```python
from build123d import *

# Parameters (mm, degrees)
BOSS_EXTRUDE1_DEPTH            = 4
SKETCH2_R                      = 2.2
BOSS_EXTRUDE2_DEPTH            = 3.5
SKETCH3_R                      = 0.75
CUT_EXTRUDE1_DEPTH             = 8.5
SKETCH4_R                      = 2.2
BOSS_EXTRUDE3_DEPTH            = 3.5
SKETCH5_R                      = 0.75
CUT_EXTRUDE2_DEPTH             = 8.5
SKETCH6_R                      = 2.2
BOSS_EXTRUDE4_DEPTH            = 3.5
SKETCH7_R                      = 0.75
CUT_EXTRUDE3_DEPTH             = 8.5
SKETCH8_R                      = 2.2
BOSS_EXTRUDE5_DEPTH            = 3.5
SKETCH9_R                      = 0.75
CUT_EXTRUDE4_DEPTH             = 8.5
SKETCH10_W                     = 20
SKETCH10_H                     = 5
BOSS_EXTRUDE6_DEPTH            = 3.5
SKETCH11_R                     = 1.5
CUT_EXTRUDE5_DEPTH             = 8.5
BOSS_EXTRUDE8_DEPTH            = 5
CBORE_FOR_M3_SHCS1_D           = 3.4
CBORE_FOR_M3_SHCS1_CBORE_D     = 6.5
CBORE_FOR_M3_SHCS1_CBORE_DEPTH = 3
FILLET1_R                      = 5
FILLET2_R                      = 3


with BuildPart() as part:
    # Sketch1 → Boss-Extrude1 (new body)
    with BuildSketch(Plane.XY):
        with BuildLine():
            Line((0, 0), (59.790168207, -3.934842784))
            ThreePointArc((59.790168207, -3.934842784), (63.68729409, -6.932891166), (62.399590235, -11.678173352))
            Line((62.399590235, -11.678173352), (40.5, -28.758482209))
            Line((40.5, -28.758482209), (40.5, -46.843965811))
            Line((40.5, -46.843965811), (35.5, -46.843965811))
            Line((35.5, -46.843965811), (35.5, -23.843965811))
            Line((35.5, -23.843965811), (23, -23.843965811))
            Line((23, -23.843965811), (23, -9.315581275))
            Line((23, -9.315581275), (-23, -9.315581275))
            Line((-23, -9.315581275), (-23, -23.843965815))
            Line((-23, -23.843965815), (-30, -23.843965815))
            Line((-30, -23.843965815), (-30, -23.624609813))
            ThreePointArc((-30, -23.624609813), (-33.311090065, -15.630931272), (-41.304768605, -12.319841207))
            Line((-41.304768605, -12.319841207), (-57, -12.319841207))
            ThreePointArc((-57, -12.319841207), (-60.975796988, -8.36893525), (-57.049937893, -4.368404043))
            Line((-57.049937893, -4.368404043), (0, 0))
        make_face()
    extrude(amount=BOSS_EXTRUDE1_DEPTH)

    # Sketch2 → Boss-Extrude2 (add)
    with BuildSketch(Plane.XY.offset(4)):
        with Locations((59.5, -8.343965811)):
            Circle(SKETCH2_R)
    extrude(amount=BOSS_EXTRUDE2_DEPTH)

    # Sketch3 → Cut-Extrude1 (cut, through all)
    with BuildSketch(Plane.XY.offset(7.5)):
        with Locations((59.5, -8.343965811)):
            Circle(SKETCH3_R)
    extrude(amount=-CUT_EXTRUDE1_DEPTH, mode=Mode.SUBTRACT)

    # Sketch4 → Boss-Extrude3 (add)
    with BuildSketch(Plane.XY.offset(4)):
        with Locations((29.5, -19.343965811)):
            Circle(SKETCH4_R)
    extrude(amount=BOSS_EXTRUDE3_DEPTH)

    # Sketch5 → Cut-Extrude2 (cut, through all)
    with BuildSketch(Plane.XY.offset(7.5)):
        with Locations((29.5, -19.343965811)):
            Circle(SKETCH5_R)
    extrude(amount=-CUT_EXTRUDE2_DEPTH, mode=Mode.SUBTRACT)

    # Sketch6 → Boss-Extrude4 (add)
    with BuildSketch(Plane.XY.offset(4)):
        with Locations((-57, -8.343965811)):
            Circle(SKETCH6_R)
    extrude(amount=BOSS_EXTRUDE4_DEPTH)

    # Sketch7 → Cut-Extrude3 (cut, through all)
    with BuildSketch(Plane.XY.offset(7.5)):
        with Locations((-57, -8.343965811)):
            Circle(SKETCH7_R)
    extrude(amount=-CUT_EXTRUDE3_DEPTH, mode=Mode.SUBTRACT)

    # Sketch8 → Boss-Extrude5 (add)
    with BuildSketch(Plane.XY.offset(4)):
        with Locations((-27, -19.343965811)):
            Circle(SKETCH8_R)
    extrude(amount=BOSS_EXTRUDE5_DEPTH)

    # Sketch9 → Cut-Extrude4 (cut, through all)
    with BuildSketch(Plane.XY.offset(7.5)):
        with Locations((-27, -19.343965811)):
            Circle(SKETCH9_R)
    extrude(amount=-CUT_EXTRUDE4_DEPTH, mode=Mode.SUBTRACT)

    # Sketch10 → Boss-Extrude6 (add)
    with BuildSketch(Plane.XY.offset(4)):
        with Locations((0, -5.399210768)):
            Rectangle(SKETCH10_W, SKETCH10_H)
    extrude(amount=BOSS_EXTRUDE6_DEPTH)

    # Sketch11 → Cut-Extrude5 (cut, through all)
    with BuildSketch(Plane.XY.offset(7.5)):
        with Locations((-7.5, -5.399210768)):
            Circle(SKETCH11_R)
        with Locations((7.5, -5.399210768)):
            Circle(SKETCH11_R)
    extrude(amount=-CUT_EXTRUDE5_DEPTH, mode=Mode.SUBTRACT)

    # Sketch12 → Boss-Extrude8 (add)
    with BuildSketch(Plane(origin=(40.5, 0, 0), x_dir=(0, 0, -1), z_dir=(1, 0, 0))):
        with BuildLine():
            ThreePointArc((-4, -29.597999119), (-6.613538808, -28.293090617), (-9.5, -27.843965811))
            Line((-9.5, -27.843965811), (-9.5, -46.843965811))
            ThreePointArc((-9.5, -46.843965811), (-6.613538808, -46.394841006), (-4, -45.089932504))
            Line((-4, -45.089932504), (-4, -29.597999119))
        make_face()
        with BuildLine():
            Line((-4, -27.843965811), (-9.5, -27.843965811))
            ThreePointArc((-9.5, -27.843965811), (-6.613538808, -28.293090617), (-4, -29.597999119))
            Line((-4, -29.597999119), (-4, -27.843965811))
        make_face()
        with BuildLine():
            Line((-9.5, -46.843965811), (-9.5, -27.843965811))
            ThreePointArc((-9.5, -27.843965811), (-19, -37.343965811), (-9.5, -46.843965811))
        make_face()
        with BuildLine():
            ThreePointArc((-4, -45.089932504), (-6.613538808, -46.394841006), (-9.5, -46.843965811))
            Line((-9.5, -46.843965811), (-4, -46.843965811))
            Line((-4, -46.843965811), (-4, -45.089932504))
        make_face()
        with BuildLine():
            ThreePointArc((0, -37.343965811), (-1.059028492, -32.985066868), (-4, -29.597999119))
            Line((-4, -29.597999119), (-4, -45.089932504))
            ThreePointArc((-4, -45.089932504), (-1.059028492, -41.702864755), (0, -37.343965811))
        make_face()
    extrude(amount=-BOSS_EXTRUDE8_DEPTH)

    # CBORE for M3 SHCS1 (through all)
    with Locations(Plane(origin=(40.5, -32.843965811, 14), x_dir=(0, 0, 1), z_dir=(1, 0, 0))):
        with Locations((0, 0), (-9, 0), (0, 9), (-9, 9)):
            CounterBoreHole(CBORE_FOR_M3_SHCS1_D / 2, CBORE_FOR_M3_SHCS1_CBORE_D / 2, CBORE_FOR_M3_SHCS1_CBORE_DEPTH)

    # Fillet1
    fillet1_edges = [part.edges().sort_by_distance(p)[0] for p in [
        (23, -9.315581275, 2),
        (-23, -9.315581275, 2),
    ]]
    fillet(fillet1_edges, radius=FILLET1_R)

    # Fillet2
    fillet2_edges = [part.edges().sort_by_distance(p)[0] for p in [
        (-30, -23.843965815, 2),
        (23, -23.843965811, 2),
        (-23, -23.843965815, 2),
    ]]
    fillet(fillet2_edges, radius=FILLET2_R)


solid = part.part
```
Part model, mm, in its own coordinate system. A direction names the side the tool comes from. Coordinates: 2 decimals unless noted, no trailing zeros. Order: outer loops, then holes, each group sorted by start corner. A loop starts at its lowest first (then second) coordinate and runs counter-clockwise, first axis right, second up. Notation, with made-up numbers: (64, 32.5) - (81, 32.5) arc R34 ccw to (81, 62.5) - close; hole circle Ø5 at (3, -32). An arc over 180 degrees is marked (long way). Return JSON: item names as keys, results as strings. Group by question number.
Item 1: Cut at A-A (x = 7.5). List the corners of the cut face in (y, z).
Item 2: Cut at B-B (y = -15.5). List the corners of the cut face in (x, z).
Item 3: Pull direction X, two halves, no side cores. Call faces 6 (the face through (-28.924, -2.215, 1.972)), 7 (the face through (63.66, -6.86, 1.97)), 8 (the face through (27.879, -17.857, 5.726)): pulls with the +X half, pulls with the -X half, needs draft (parallel to the pull), parting line crosses it, or undercut.
Item 4: Cut at C-C (x = -46.5). List the corners of the cut face in (y, z).
Item 5: Drill centre lines: probe 1 along Y at (x, z) = (38.9, 5); probe 2 along X at (y, z) = (-19.5, 6.75); probe 3 along X at (y, z) = (-8, 1). Where is each one in solid material? Low to high. Write a range as from..to.
Item 6: Which spindle directions (+Z, -Z, +X, -X, +Y, -Y) get a long thin tool onto all of the face, cutting with end or side? Do faces 1 (the face through (0, -7.899, 6)), 2 (the face through (0, -9.316, 2)), 3 (the face through (10, -5, 6)), 4 (the face through (-28.621, -17.857, 5.726)), 5 (the face through (39.02, -33.82, 8.1)). Say none if no direction does.
Item 7: Pin check, flat tips, straight feed: pin 1 (1 mm diameter, centred on x = -27.5, y = -12.5, fed in from +Z); pin 2 (2 mm diameter, centred on y = -17.5, z = 1.5, fed in from -X); pin 3 (10.5 mm diameter, centred on y = -41.84, z = 14, fed in from +X); pin 4 (1.4 mm diameter, centred on x = 29.5, y = -19.34, fed in from -Z). Stop position of each tip, or through.
Check values:
{
 "1": {"outline": "(-9.32, 0) - (-6.9, 0) - (-6.9, 7.5) - (-7.9, 7.5) - (-7.9, 4) - (-9.32, 4) - close; (-3.9, 0) - (-0.49, 0) - (-0.49, 4) - (-2.9, 4) - (-2.9, 7.5) - (-3.9, 7.5) - close"},
 "2": {"outline": "(-33.44, 0) - (-23, 0) - (-23, 4) - (-33.44, 4) - close; (23, 0) - (57.5, 0) - (57.5, 4) - (23, 4) - close"},
 "3": {"face 6": "pulls with the -X half", "face 7": "pulls with the +X half", "face 8": "undercut"},
 "4": {"outline": "(-12.32, 0) - (-3.56, 0) - (-3.56, 4) - (-12.32, 4) - close"},
 "5": {"probe 1": "y = -46.84..-45.09, -38.59..-36.09, -29.59..-27.84", "probe 2": "x = -29.19..-27.73, -26.27..-24.81, 27.31..28.77, 30.23..31.69", "probe 3": "x = -60.96..-57.67, -56.33..58.83, 60.17..63.91"},
 "6": {"face 1": "+Z, -Y", "face 2": "+Z, -Z, -Y", "face 3": "+Z, +Y, -Y", "face 4": "+Z", "face 5": "+X"},
 "7": {"pin 1": "stops at z = 4", "pin 2": "stops at x = -32.53", "pin 3": "stops at x = 40.5", "pin 4": "passes through"}
}
